Geometry: final body of the model. Coordinates: model frame, mm. Face numbers are marked on the shaded views. A direction names the side the tool comes from. Coordinates: 2 decimals unless noted, no trailing zeros. Loops run counter-clockwise (first coordinate to the right, second up) from the corner with the lowest first, then second, coordinate; pieces in that order, holes last. Notation, with made-up numbers: (-30, 41) -> (13, 41) arc R34 ccw to (13, 73) -> close; hole circle Ø9 at (12.5, 29.25). An arc over 180 degrees is marked (long way). One line per item, written item: value. Start each with the question number.
Item 1: Set-up query: the marked faces 1 and 2. Return all of +Z, -Z, +X, -X, +Y, -Y with unobstructed straight access to the full face (end or side cutting, diameter ignored); none if empty.
Item 2: Mould query, pull axis X, two halves, no side actions, for the marked faces 3 and 4. Classes: +X half, -X half, draft (parallel to the pull), parting line (faces both ways), or undercut.
Item 3: Section query B-B on x = 8.5. Return loops of the section in (y, z), then the cut area to 3 significant figures.
Item 4: Contact query for flat-ended pins moving along their axis: pin 1 Ø6 at (x, z) = (-18, 6.5) entering from -Y; pin 2 Ø9 at (y, z) = (8, 12) entering from -X; pin 3 Ø8 at (x, z) = (6.5, 9) entering from +Y. Output: stop coordinate, or through.
Item 5: Ray query, probe 1 along Z at (x, y) = (1, -9.5); probe 2 along X at (y, z) = (-10.5, 9); probe 3 along X at (y, z) = (-3.5, 14). Return the intervals inside material, ascending. Write a range as from..to.
Item 6: Section query A-A on z = 8. Return loops of the section in (x, y), then the cut area to 3 significant figures.
Item 7: Section query D-D on z = 2. Return loops of the section in (x, y), then the cut area to 3 significant figures.
Item 8: Section query C-C on y = 2. Return loops of the section in (x, z).
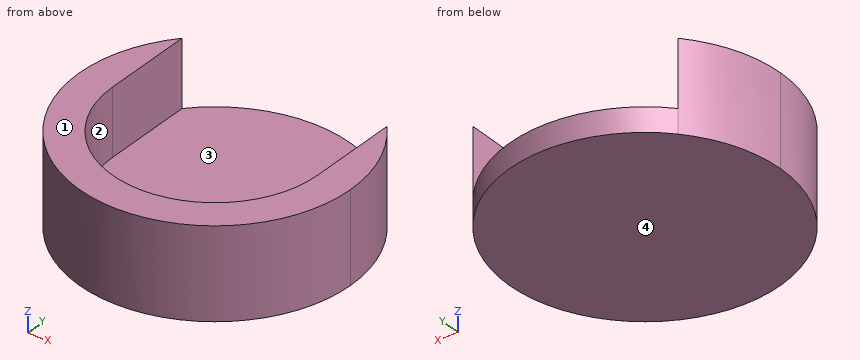
from build123d import *

# Parameters (mm, degrees)
F1_DEPTH = 15
F2_DEPTH = 4


# Not quite as in the source:
# - a feature names something its author has since deleted; it is built from what else it names


with BuildPart() as f1:
    # F0 (on Top) → F1 (new body)
    with BuildSketch(Plane.XY):
        with BuildLine():
            Line((22.5, 0), (17, 0))
            ThreePointArc((17, 0), (0, -17), (-17, 0))
            Line((-17, 0), (-22.5, 0))
            ThreePointArc((-22.5, 0), (0, -22.5), (22.5, 0))
        make_face()
        with BuildLine():
            Line((-22.5, 0), (-17, 0))
            Line((-17, 0), (-17, 14.739402973))
            ThreePointArc((-17, 14.739402973), (-21.0802039838, 7.8660663613), (-22.5, 0))
        make_face()
        with BuildLine():
            Line((17, 14.739402973), (17, 0))
            Line((17, 0), (22.5, 0))
            ThreePointArc((22.5, 0), (21.0802039838, 7.8660663613), (17, 14.739402973))
        make_face()
    extrude(amount=F1_DEPTH)

    # F0 (on Top) → F2 (join)
    with BuildSketch(Plane.XY):
        with BuildLine():
            Line((-17, 0), (17, 0))
            ThreePointArc((17, 0), (0, 17), (-17, 0))
        make_face()
        with BuildLine():
            ThreePointArc((-17, 0), (0, -17), (17, 0))
            Line((17, 0), (-17, 0))
        make_face()
        with BuildLine():
            ThreePointArc((-17, 0), (0, 17), (17, 0))
            Line((17, 0), (17, 14.739402973))
            ThreePointArc((17, 14.739402973), (0, 22.5), (-17, 14.739402973))
            Line((-17, 14.739402973), (-17, 0))
        make_face()
    extrude(amount=F2_DEPTH)


solid = f1.part
Reply:
1. face 1: +Z, +X, -X, +Y, -Y
1. face 2: +Z, +Y
2. face 3: undercut
2. face 4: draft
3. outline: (-20.83, 0) -> (20.83, 0) -> (20.83, 4) -> (-14.72, 4) -> (-14.72, 15) -> (-20.83, 15) -> close
3. area: 234 mm²
4. pin 1: stops at y = -16.77
4. pin 2: stops at x = -22.23
4. pin 3: stops at y = -13.37
5. probe 1: z = 0..4
5. probe 2: x = -19.9..-13.37, 13.37..19.9
5. probe 3: x = -22.23..-16.64, 16.64..22.23
6. outline: (-17, 0) -> (-17, 14.74) arc R22.5 ccw (long way) to (17, 14.74) -> (17, 0) arc R17 cw to start
6. area: 452 mm²
7. outline: circle Ø45 at (0, 0)
7. area: 1,590 mm²
8. outline: (-22.41, 0) -> (22.41, 0) -> (22.41, 15) -> (17, 15) -> (17, 4) -> (-17, 4) -> (-17, 15) -> (-22.41, 15) -> close
